from build123d import *

# Parameters (mm, degrees)
PAD006_DEPTH    = 7
POCKET003_DEPTH = 6.001
POCKET004_DEPTH = 12
POCKET005_DEPTH = 2


with BuildPart() as part:
    # Sketch008 → Pad006 (new body)
    with BuildSketch(Plane.XY):
        with BuildLine():
            ThreePointArc((6.40542, -26.743608), (27.5, 0), (6.40542, 26.743608))
            Line((6.40542, 26.743608), (6, 26.743608))
            Line((6, 26.743608), (6, -26.743608))
            Line((6, -26.743608), (6.40542, -26.743608))
        make_face()
    extrude(amount=PAD006_DEPTH)

    # Sketch009 → Pocket003 (cut, through all)
    with BuildSketch(Plane.XY.offset(1)):
        with BuildLine():
            Line((9.069885, 20.990567), (9.069885, 12.381273))
            Line((6.8, 12.381273), (9.069885, 12.381273))
            Line((6.8, -12.097779), (6.8, 12.381273))
            Line((9.069885, -12.097779), (6.8, -12.097779))
            Line((9.069885, -12.097779), (9.069885, -18.131377))
            Line((9.069885, -18.131377), (11.681826, -21.861614))
            ThreePointArc((11.681826, -21.861614), (17.167285, -17.940734), (21.270115, -12.59))
            Line((23.54, -12.59), (21.270115, -12.59))
            Line((23.54, 12.59), (23.54, -12.59))
            Line((21.270115, 12.59), (23.54, 12.59))
            ThreePointArc((21.270115, 12.59), (18.415103, 17.190589), (14.558075, 20.990567))
            Line((9.069885, 20.990567), (14.558075, 20.990567))
        make_face()
    extrude(amount=POCKET003_DEPTH, mode=Mode.SUBTRACT)

    # Sketch010 → Pocket004 (cut)
    with BuildSketch(Plane(origin=(25, 25, 0), x_dir=(-0.5, 0.866025, 0), z_dir=(0.866025, 0.5, 0))):
        with BuildLine():
            ThreePointArc((-1.06066, 4.96066), (0, 2.4), (1.06066, 4.96066))
            Line((0.62132, 5.4), (1.06066, 4.96066))
            Line((-0.62132, 5.4), (0.62132, 5.4))
            Line((-1.06066, 4.96066), (-0.62132, 5.4))
        make_face()
    extrude(amount=-POCKET004_DEPTH, mode=Mode.SUBTRACT)

    # Sketch011 → Pocket005 (cut)
    with BuildSketch(Plane.XY.offset(7)):
        Polygon((9.546117, -17.484219), (3.82131, -19.595547), (3.82131, -24.962748), (5.727243, -24.812279), (8.868557, -24.025229), (11.914429, -21.802042), align=None)
    extrude(amount=-POCKET005_DEPTH, mode=Mode.SUBTRACT)


solid = part.part
Source: CAD feature listing. Evaluate the final solid. Frame: model axes, mm. A direction names the side the tool comes from. Give positions to 0.01 mm unless a question says otherwise; leave off trailing zeros. Write each loop counter-clockwise with the first axis right and the second up, starting at its lowest first coordinate (ties: lowest second). Pieces come first, ordered by that corner, then holes. Notation, with made-up numbers: M 66,-38.5 L 111,-38.5 A18 ccw 111,-27.5 Z; hole C 56,-19 d9. An arc over 180 degrees is marked long. Return JSON: item names as keys, results as strings. Group by question number.
1) Set-up query: faces 5 (the face through (6.8, 0, 4)), 6 (the face through (7.41, -24.39, 6.01)), 7 (the face through (17.601, 19.753, 5.177)), 8 (the face through (14, 0, 0)). Return all of +Z, -Z, +X, -X, +Y, -Y with unobstructed straight access to the full face (end or side cutting, diameter ignored); none if empty.
2) Cut plane B-B, the plane z = 3.75. Output: boundary loops of the cut face in (x, y), then the cut area to 3 significant figures.
3) Cut plane A-A, the plane x = 22. Output: boundary loops of the cut face in (y, z), then the cut area to 3 significant figures.
4) Cut plane D-D, the plane x = 10.5. Output: boundary loops of the cut face in (y, z), then the cut area to 3 significant figures.
5) Draft query along Y for faces 1 (the face through (27.495, -0.514, 3.451)), 2 (the face through (17.099, -18.006, 3.958)), 3 (the face through (10.37, -22.93, 6.01)), 4 (the face through (24, 4, 7)). Return one class per face: released by +Y, released by -Y, zero draft, split by the parting line, or undercut.
6) First-contact query: pin 1 Ø1.8 at (x, z) = (22, 5) entering from -Y; pin 2 Ø2.5 at (x, z) = (22.5, 5) entering from +Y; pin 3 Ø1.1 at (x, z) = (8, 5) entering from +Y. Flat tips, straight axial feed; report the tip coordinate or a pass-through.
7) Ray query, L1, parallel to Z at x = 8.75, y = 4.5; L2, parallel to Y at x = 18.5, z = 3.5; L3, parallel to Y at x = 9.75, z = 5.25. Return the intervals inside material, ascending.
8) Cut plane C-C, the plane y = -13.5. Output: boundary loops of the cut face in (x, z), then the cut area to 3 significant figures.
Data:
{
 "1": {"face 5": "+Z", "face 6": "+Z, -X", "face 7": "none", "face 8": "-Z, +X, -X, +Y, -Y"},
 "2": {"outline": "M 6,-26.74 L 6.41,-26.74 A27.5 ccw 19.04,19.84 L 17.09,18.71 A22.86 cw 21.27,12.59 L 23.54,12.59 L 23.54,-12.59 L 21.27,-12.59 A22.86 cw 11.68,-21.86 L 9.07,-18.13 L 9.07,-12.1 L 6.8,-12.1 L 6.8,12.38 L 9.07,12.38 L 9.07,20.99 L 14.56,20.99 A22.86 cw 14.78,20.82 L 16.64,21.9 A27.5 ccw 6.41,26.74 L 6,26.74 Z", "area": "282 mm²"},
 "3": {"outline": "M -16.5,0 L 16.5,0 L 16.5,7 L 12.59,7 L 12.59,1 L -12.59,1 L -12.59,7 L -16.5,7 Z", "area": "79.9 mm²"},
 "4": {"outline": "M -25.42,0 L 25.42,0 L 25.42,7 L 20.99,7 L 20.99,1 L -20.17,1 L -20.17,5 L -22.83,5 L -22.83,7 L -25.42,7 Z", "area": "104 mm²"},
 "5": {"face 1": "split by the parting line", "face 2": "undercut", "face 3": "undercut", "face 4": "zero draft"},
 "6": {"pin 1": "stops at y = -17.64", "pin 2": "stops at y = 17.46", "pin 3": "stops at y = 26.47"},
 "7": {"L1": "z = 0 to 1", "L2": "y = -20.35 to -16.54, 17.08 to 19.58", "L3": "y = -25.71 to -23.38, 20.99 to 25.71"},
 "8": {"outline": "M 6,0 L 23.96,0 L 23.96,7 L 20.74,7 L 20.74,1 L 9.07,1 L 9.07,7 L 6,7 Z", "area": "55.7 mm²"}
}
